Source: CAD feature listing. Evaluate the final solid. Frame: model axes, mm. Face numbers are marked on the shaded views. A direction names the side the tool comes from. Give positions to 0.01 mm unless a question says otherwise; leave off trailing zeros. Order: outer loops, then holes, each group sorted by start corner. A loop starts at its lowest first (then second) coordinate and runs counter-clockwise, first axis right, second up. Notation, with made-up numbers: M 15,-3.75 L 24,-3.75 A19 ccw 24,24.25 Z; hole C -5.75,-15.75 d8. An arc over 180 degrees is marked long. Use CSV: the item, a comma, the result in double quotes. Start each with the question number.
1. Section query B-B, the plane y = -22. Return the cut outline in (x, z) (3 decimals).
2. Section query C-C, the plane z = 0. Return the cut outline in (x, y) (3 decimals), plus the area to 3 significant figures.
3. Pin query (flat end, axial travel): P1, Ø2, axis at x = 60.5, z = 3.5, coming from the +Y side; P2, Ø18.5, axis at x = 54.5, z = 2, coming from the -Y side; P3, Ø10, axis at y = 0, z = -14, coming from the -X side. Return the tip coordinate at first contact, or that it passes through.
4. Section query D-D, the plane y = -1. Return the cut outline in (x, z) (3 decimals).
5. Line query: line 1 along Z through (x, y) = (0, 10) (3 decimals); line 2 along X through (y, z) = (-5.5, -5.5); line 3 along Z through (x, y) = (5.5, -7.5). Output: solid intervals per line, ascending. Write a range as [from, to].
6. Reachability of the marked faces 4, 5 and 6 from +Z, -Z, +X, -X, +Y, -Y: full face, straight path, thin tool, end or side. Return the list, or none.
7. Mould query, pull axis X, two halves, no side actions, for the marked faces 1, 2 and 3. Classes: released by +X, released by -X, zero draft, split by the parting line, or undercut.
8. Section query A-A, the plane x = 0. Return the cut outline in (y, z) (3 decimals).
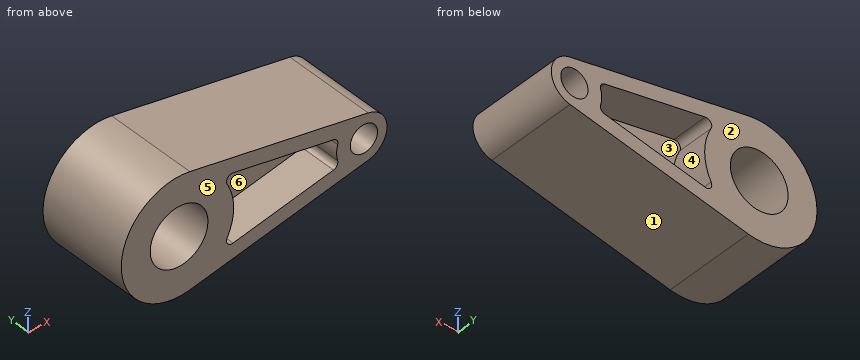
from build123d import *

# Parameters (mm, degrees)
F1_DEPTH = 25
F3_D     = 15
F4_R     = 15.875
F5_DEPTH = 50.001
F7_DEPTH = 20
F9_DEPTH = 20
F10_R    = 3
F11_R    = 3


with BuildPart() as f1:
    # F0 (on Front) → F1 (new body, symmetric)
    with BuildSketch(Plane.XZ):
        with BuildLine():
            Line((103.98125, 12.47476), (5.953125, 31.186901))
            ThreePointArc((5.953125, 31.186901), (-31.75, 0), (5.953125, -31.186901))
            Line((5.953125, -31.186901), (103.98125, -12.47476))
            ThreePointArc((103.98125, -12.47476), (114.3, 0), (103.98125, 12.47476))
        make_face()
    extrude(amount=F1_DEPTH, both=True)

    # F3 (through all)
    with Locations(Plane.XZ.offset(25)):
        with Locations((101.6, 0)):
            Hole(F3_D / 2)

    # F4 (on face) → F5 (cut, through all)
    with BuildSketch(Plane.XZ.offset(25)):
        Circle(F4_R)
    extrude(amount=-F5_DEPTH, mode=Mode.SUBTRACT)

    # F6 (on face) → F7 (cut)
    with BuildSketch(Plane.XZ.offset(25)):
        with BuildLine():
            Line((88.489236, 7.287515), (22.456658, 19.892172))
            ThreePointArc((22.456658, 19.892172), (30, 0), (22.456658, -19.892172))
            Line((22.456658, -19.892172), (88.489236, -7.287515))
            ThreePointArc((88.489236, -7.287515), (86.6, 0), (88.489236, 7.287515))
        make_face()
    extrude(amount=-F7_DEPTH, mode=Mode.SUBTRACT)

    # F8 (on face) → F9 (cut)
    with BuildSketch(Plane(origin=(0, 25, 0), x_dir=(-1, 0, 0), z_dir=(0, 1, 0))):
        with BuildLine():
            Line((-88.489236, -7.287515), (-22.456658, -19.892172))
            ThreePointArc((-22.456658, -19.892172), (-30, 0), (-22.456658, 19.892172))
            Line((-22.456658, 19.892172), (-88.489236, 7.287515))
            ThreePointArc((-88.489236, 7.287515), (-86.6, 0), (-88.489236, -7.287515))
        make_face()
    extrude(amount=-F9_DEPTH, mode=Mode.SUBTRACT)

    # F10
    f10_edges = [f1.edges().sort_by_distance(p)[0] for p in [
        (22.456658, -15, -19.892172),
        (22.456658, -15, 19.892172),
        (22.456658, 15, 19.892172),
        (22.456658, 15, -19.892172),
    ]]
    fillet(f10_edges, radius=F10_R)

    # F11
    f11_edges = [f1.edges().sort_by_distance(p)[0] for p in [
        (88.489236, 15, -7.287515),
        (88.489236, 15, 7.287515),
        (88.489236, -15, 7.287515),
        (88.489236, -15, -7.287515),
    ]]
    fillet(f11_edges, radius=F11_R)


solid = f1.part
Result set:
1,outline,"M 5.953,-31.187 L 103.981,-12.475 A12.7 ccw 103.981,12.475 L 5.953,31.187 A31.75 ccw long Z; hole C 0,0 d31.75; hole M 26.451,-14.155 A3 ccw 29.658,-18.518 L 84.88,-7.977 A3 ccw 87.198,-4.191 A15 cw 87.198,4.191 A3 ccw 84.88,7.977 L 29.658,18.518 A3 ccw 26.451,14.155 A30 cw Z; hole C 101.6,0 d15"
2,outline,"M -31.75,-25 L -15.875,-25 L -15.875,25 L -31.75,25 Z; M 15.875,-25 L 30,-25 L 30,-5 L 86.6,-5 L 86.6,-25 L 94.1,-25 L 94.1,25 L 86.6,25 L 86.6,5 L 30,5 L 30,25 L 15.875,25 Z; M 109.1,-25 L 114.3,-25 L 114.3,25 L 109.1,25 Z"
2,area,"2,700 mm2"
3,P1,"y = 5"
3,P2,"y = -5"
3,P3,"x = -30.45"
4,outline,"M 5.953,-31.187 L 103.981,-12.475 A12.7 ccw 103.981,12.475 L 5.953,31.187 A31.75 ccw long Z; hole C 0,0 d31.75; hole C 101.6,0 d15"
5,line 1,"[-31.75, -15.875], [15.875, 31.75]"
5,line 2,"[-31.27, -14.89], [14.89, 29.49], [87.28, 96.5], [106.7, 113.05]"
5,line 3,"[-31.27, -14.89], [14.89, 31.27]"
6,face 4,"+Y"
6,face 5,"+Z, -Z, +X, -X, -Y"
6,face 6,"-Y"
7,face 1,"released by +X"
7,face 2,"zero draft"
7,face 3,"undercut"
8,outline,"M -25,-31.75 L 25,-31.75 L 25,-15.875 L -25,-15.875 Z; M -25,15.875 L 25,15.875 L 25,31.75 L -25,31.75 Z"
